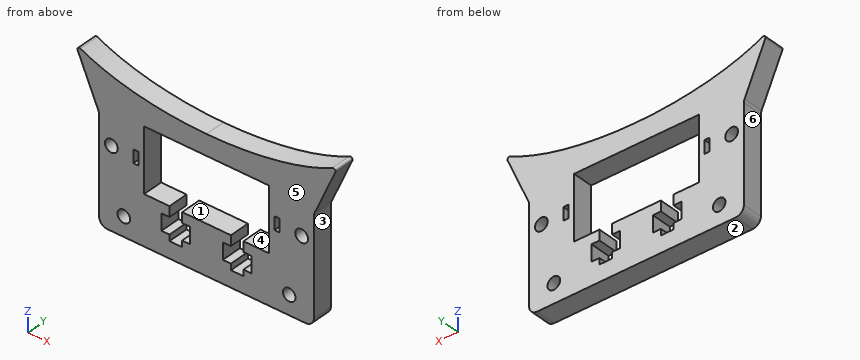
```python
from build123d import *

# Parameters (mm, degrees)
SKETCH1_W           = 105
SKETCH1_H           = 65
BOSS_EXTRUDE1_DEPTH = 10
SKETCH2_W           = 61
SKETCH2_H           = 31
CUT_EXTRUDE1_DEPTH  = 11
SKETCH3_W           = 6.15
SKETCH3_H           = 5
SKETCH3_H_2         = 3
CUT_EXTRUDE2_DEPTH  = 10
SKETCH4_R           = 3.125
SKETCH4_W           = 2.5
SKETCH4_H           = 6.35
CUT_EXTRUDE3_DEPTH  = 11
BOSS_EXTRUDE2_DEPTH = 10
SKETCH6_R           = 3.075
CUT_EXTRUDE4_DEPTH  = 11.0000001
FILLET2_R           = 1
FILLET1_R           = 4


with BuildPart() as part:
    # Sketch1 → Boss-Extrude1 (new body)
    with BuildSketch(Plane(origin=(0, 0, 0), x_dir=(1, 0, 0), z_dir=(0, 1, 0))):
        Rectangle(SKETCH1_W, SKETCH1_H)
    extrude(amount=BOSS_EXTRUDE1_DEPTH)

    # Sketch2 → Cut-Extrude1 (cut, through all)
    with BuildSketch(Plane(origin=(0, 10, 0), x_dir=(1, 0, 0), z_dir=(0, 1, 0))):
        with Locations((0, -7)):
            Rectangle(SKETCH2_W, SKETCH2_H)
    extrude(amount=-CUT_EXTRUDE1_DEPTH, mode=Mode.SUBTRACT)

    # Sketch3 → Cut-Extrude2 (cut)
    with BuildSketch(Plane(origin=(0, 10, 0), x_dir=(1, 0, 0), z_dir=(0, 1, 0))):
        with Locations((-15, 11)):
            Rectangle(SKETCH3_W, SKETCH3_H)
        Polygon((-18.075, 21.5), (-22, 21.5), (-22, 13.5), (-18.075, 13.5), (-11.925, 13.5), (-8, 13.5), (-8, 21.5), (-11.925, 21.5), (-11.925, 18.5), (-18.075, 18.5), align=None)
        with Locations((-15, 20)):
            Rectangle(SKETCH3_W, SKETCH3_H_2)
        with Locations((-15, 23)):
            Rectangle(SKETCH3_W, SKETCH3_H_2)
    cut_extrude2 = extrude(amount=-CUT_EXTRUDE2_DEPTH, mode=Mode.SUBTRACT)

    # Sketch4 → Cut-Extrude3 (cut, through all)
    with BuildSketch(Plane(origin=(0, 10, 0), x_dir=(1, 0, 0), z_dir=(0, 1, 0))):
        with Locations((-46.5, -6.5)):
            Circle(SKETCH4_R)
        with Locations((-34.5, -6.5)):
            Rectangle(SKETCH4_W, SKETCH4_H)
    cut_extrude3 = extrude(amount=-CUT_EXTRUDE3_DEPTH, mode=Mode.SUBTRACT)

    # Sketch5 → Boss-Extrude2 (add)
    with BuildSketch(Plane(origin=(0, 0, 0), x_dir=(1, 0, 0), z_dir=(0, 1, 0))):
        with BuildLine():
            Line((0, -32.5), (-52.5, -19.039128985))
            Line((-52.5, -19.039128985), (-64.119998298, -45.565168911))
            add(Edge.make_bspline(
                [(0, -32.5), (-40.125285882, -32.5), (-64.119998298, -45.565168911)],
                knots=[4.71238898, 4.71238898, 4.71238898, 5.642188346, 5.642188346, 5.642188346], degree=2, weights=[1, 0.893866546, 1]))
        make_face()
    boss_extrude2 = extrude(amount=BOSS_EXTRUDE2_DEPTH)

    # Sketch6 → Cut-Extrude4 (cut, through all)
    with BuildSketch(Plane(origin=(0, 10, 0), x_dir=(1, 0, 0), z_dir=(0, 1, 0))):
        with Locations((-40.420875644, 23.095045258)):
            Circle(SKETCH6_R)
    cut_extrude4 = extrude(amount=-CUT_EXTRUDE4_DEPTH, mode=Mode.SUBTRACT)

    # Mirror1: Cut-Extrude2, Cut-Extrude3, Boss-Extrude2, Cut-Extrude4 across plane
    add(cut_extrude2.mirror(Plane(origin=(0, 0, 0), x_dir=(0, 0, 1), z_dir=(1, 0, 0))), mode=Mode.SUBTRACT)
    add(cut_extrude3.mirror(Plane(origin=(0, 0, 0), x_dir=(0, 0, 1), z_dir=(1, 0, 0))), mode=Mode.SUBTRACT)
    add(boss_extrude2.mirror(Plane(origin=(0, 0, 0), x_dir=(0, 0, 1), z_dir=(1, 0, 0))))
    add(cut_extrude4.mirror(Plane(origin=(0, 0, 0), x_dir=(0, 0, 1), z_dir=(1, 0, 0))), mode=Mode.SUBTRACT)

    # Fillet2
    fillet2_edges = [part.edges().sort_by_distance(p)[0] for p in [
        (-64.119998298, 5, 45.565168911),
        (64.119998298, 5, 45.565168911),
    ]]
    fillet(fillet2_edges, radius=FILLET2_R)

    # Fillet1
    fillet1_edges = [part.edges().sort_by_distance(p)[0] for p in [
        (52.5, 5, 19.039128985),
        (-52.5, 5, -32.5),
        (52.5, 5, -32.5),
        (-52.5, 5, 19.039128985),
    ]]
    fillet(fillet1_edges, radius=FILLET1_R)


solid = part.part
```
Read the model definition and answer for the solid it produces. Units are mm, in the model's axes. Face numbers are marked on the shaded views. A direction names the side the tool comes from. Round coordinates to 2 decimals unless told otherwise and drop trailing zeros. Loops run counter-clockwise (first coordinate to the right, second up) from the corner with the lowest first, then second, coordinate; pieces in that order, holes last. Notation, with made-up numbers: (33, -14) -> (66, -14) arc R19 ccw to (66, 0) -> close; hole circle Ø9 at (-18, 75). An arc over 180 degrees is marked (long way). One line per item, written item: value.
1) A cutting plane is placed at B-B (y = 2.5). Give the number of separate pieces and of enclosed holes in the cut face, and give its area (3 significant figures).
Answer list:
separate pieces: 1
enclosed holes: 7
area: 4,960 mm²
2) Flat-ended cylindrical pins translate along their axes: P1, Ø5.5, axis at y = 4.5, z = -10, coming from the +X side; P2, Ø12, axis at x = -27, z = -16, coming from the -Y side; P3, Ø2.5, axis at y = 5.5, z = -17, coming from the -X side; P4, Ø3.5, axis at x = 40.42, z = -23.1, coming from the -Y side. Find the tip coordinate at first contact, or state that the pin passes through.
Answer list:
P1: stops at x = 52.5
P2: stops at y = 0
P3: stops at x = -52.5
P4: passes through
3) The mould has two halves that part along X. Classify the marked faces 4, 5 and 6: pulls with the +X half, pulls with the -X half, needs draft (parallel to the pull), parting line crosses it, or undercut.
Answer list:
face 4: undercut
face 5: needs draft
face 6: pulls with the -X half
4) For the marked faces 1, 2 and 3, determine the directions among +Z, -Z, +X, -X, +Y, -Y from which every point of the face is accessible in a straight line to the end or side of a thin tool.
Answer list:
face 1: +Y, -Y
face 2: -Z, +X, -X, +Y, -Y
face 3: -Z, +X, +Y, -Y
5) A cutting plane is placed at A-A (z = 6.5). Determine the outline of the cut face in (x, y) (3 decimals).
Answer list:
outline: (-52.5, 0) -> (-49.625, 0) -> (-49.625, 10) -> (-52.5, 10) -> close; (-43.375, 0) -> (-35.75, 0) -> (-35.75, 10) -> (-43.375, 10) -> close; (-33.25, 0) -> (-30.5, 0) -> (-30.5, 10) -> (-33.25, 10) -> close; (30.5, 0) -> (33.25, 0) -> (33.25, 10) -> (30.5, 10) -> close; (35.75, 0) -> (43.375, 0) -> (43.375, 10) -> (35.75, 10) -> close; (49.625, 0) -> (52.5, 0) -> (52.5, 10) -> (49.625, 10) -> close
6) A cutting plane is placed at C-C (z = 29). Determine the outline of the cut face in (x, y), and give its area (3 significant figures).
Answer list:
outline: (-56.86, 0) -> (56.86, 0) -> (56.86, 10) -> (-56.86, 10) -> close
area: 1,140 mm²
7) Consider L1, parallel to X at y = 4.5, z = 6.5 (3 decimals); L2, parallel to X at y = 2, z = -17; L3, parallel to X at y = 7.25, z = 1. Determine where each line is inside the solid, lowest interval first. Write a range as [from, to].
Answer list:
L1: x = [-52.5, -49.625], [-43.375, -35.75], [-33.25, -30.5], [30.5, 33.25], [35.75, 43.375], [49.625, 52.5]
L2: x = [-52.5, -22], [-8, 8], [22, 52.5]
L3: x = [-52.5, -30.5], [30.5, 52.5]
